Design review of the part built by this model. Coordinates are the model's own, in mm. Coordinates: 2 decimals unless noted, no trailing zeros. Order: outer loops, then holes, each group sorted by start corner. A loop starts at its lowest first (then second) coordinate and runs counter-clockwise, first axis right, second up. Notation, with made-up numbers: M -7.5,0 L -2.5,0 A11 cw -2.5,10 Z; hole C 52,57.5 d10. An arc over 180 degrees is marked long. Answer in a Markdown table with one row per item.
from build123d import *

# Parameters (mm, degrees)
SKETCH1_R           = 1.5
BOSS_EXTRUDE1_DEPTH = 3


with BuildPart() as part:
    # Sketch1 → Boss-Extrude1 (new body)
    with BuildSketch(Plane(origin=(0, 0, 0), x_dir=(1, 0, 0), z_dir=(0, 1, 0))):
        with BuildLine():
            Line((0, 0), (176, 0))
            Line((176, 0), (216, -40))
            Line((216, -40), (216, -255))
            ThreePointArc((216, -255), (233, -272), (250, -255))
            Line((250, -255), (250, 259.060301809))
            ThreePointArc((250, 259.060301809), (233, 276.060301809), (216, 259.060301809))
            Line((216, 259.060301809), (216, 50))
            Line((216, 50), (0, 50))
            Line((0, 50), (0, 0))
        make_face()
        with Locations(Location((238.092169369, 265.230375643, 0), (0, 0, 270))):
            Circle(SKETCH1_R, mode=Mode.SUBTRACT)
        with Locations(Location((225.673037322, 265.107252935, 0), (0, 0, 270))):
            Circle(SKETCH1_R, mode=Mode.SUBTRACT)
        with Locations(Location((227.907830631, 252.890227975, 0), (0, 0, 270))):
            Circle(SKETCH1_R, mode=Mode.SUBTRACT)
        with Locations(Location((240.326962678, 253.013350683, 0), (0, 0, 270))):
            Circle(SKETCH1_R, mode=Mode.SUBTRACT)
        with Locations(Location((226.282485579, -248.282485579, 0), (0, 0, 270))):
            Circle(SKETCH1_R, mode=Mode.SUBTRACT)
        with Locations(Location((238.656854249, -249.343145751, 0), (0, 0, 270))):
            Circle(SKETCH1_R, mode=Mode.SUBTRACT)
        with Locations(Location((239.717514421, -261.717514421, 0), (0, 0, 270))):
            Circle(SKETCH1_R, mode=Mode.SUBTRACT)
        with Locations(Location((227.343145751, -260.656854249, 0), (0, 0, 270))):
            Circle(SKETCH1_R, mode=Mode.SUBTRACT)
        with Locations(Location((15, 25, 0), (0, 0, 270))):
            Circle(SKETCH1_R, mode=Mode.SUBTRACT)
        with Locations(Location((50, 25, 0), (0, 0, 270))):
            Circle(SKETCH1_R, mode=Mode.SUBTRACT)
    extrude(amount=BOSS_EXTRUDE1_DEPTH)


solid = part.part
(1) Add section C-C, the plane z = -88. Give the boundary of the cut face in (x, y).
Return value:
| item | result |
|---|---|
| outline | M 216,0 L 250,0 L 250,3 L 216,3 Z |
(2) Insertion check: pin 1 Ø3.5 at (x, z) = (227.34, 260.66) entering from +Y; pin 2 Ø1.8 at (x, z) = (15, -25) entering from -Y; pin 3 Ø1.5 at (x, y) = (115.5, 2) entering from -Z; pin 4 Ø0.9 at (y, z) = (1, -116) entering from -X. Each pin has a flat end and moves straight along its axis. Give the tip position at first contact, or say it passes through.
Return value:
| item | result |
|---|---|
| pin 1 | stops at y = 3 |
| pin 2 | passes through |
| pin 3 | stops at z = -50 |
| pin 4 | stops at x = 216 |
(3) Add section B-B, the plane x = 200. Give the boundary of the cut face in (y, z).
Return value:
| item | result |
|---|---|
| outline | M 0,-50 L 3,-50 L 3,24 L 0,24 Z |
(4) For line 1 along X through (y, z) = (1.3, -25); line 2 along X through (y, z) = (0.7, 205.5); line 3 along Z through (x, y) = (22, 1.35), list the stretches that pass through material, from the lowest coordinate up. Write a range as from..to.
Return value:
| item | result |
|---|---|
| line 1 | x = 0..13.5, 16.5..48.5, 51.5..250 |
| line 2 | x = 216..250 |
| line 3 | z = -50..0 |
(5) Add section A-A, the plane y = 1.9. Give the number of separate pieces and of enclosed holes in the cut face, and give its area (3 significant figures).
Return value:
| item | result |
|---|---|
| separate pieces | 1 |
| enclosed holes | 10 |
| area | 29,900 mm2 |
